Geometry: final body of the model. Coordinates: model frame, mm. Face numbers are marked on the shaded views. A direction names the side the tool comes from. Give positions to 0.01 mm unless a question says otherwise; leave off trailing zeros. Loops run counter-clockwise (first coordinate to the right, second up) from the corner with the lowest first, then second, coordinate; pieces in that order, holes last.
from build123d import *

# Parameters (mm, degrees)
BOSS_EXTRUDE1_START = 1.6
SKETCH2_R           = 4.7625
BOSS_EXTRUDE1_DEPTH = 2.3
BOSS_EXTRUDE2_START = 4.5
SKETCH5_R           = 0.846945363
BOSS_EXTRUDE2_DEPTH = 1
SKETCH6_R           = 0.645187132
CUT_EXTRUDE1_DEPTH  = 5
SKETCH9_W           = 0.137399245
SKETCH9_H           = 0.594121804
BOSS_EXTRUDE3_DEPTH = 3
SKETCH11_R          = 0.94402027
CUT_EXTRUDE2_DEPTH  = 3
SKETCH13_R          = 0.99938664
SKETCH13_R_2        = 0.759397748
CUT_EXTRUDE4_DEPTH  = 4


with BuildPart() as part:
    # Sketch1 → Revolve1 (revolve)
    with BuildSketch(Plane.XY):
        Polygon((0, 7.249356935), (-2.68096621, 7.249356935), (-2.68096621, 0), (-4.484856827, 0), (-4.484856827, 10.8), (-4.7625, 10.8), (-4.7625, 0), (-6.35, 0), (-6.35, -1.2), (-4.7625, -1.2), (-4.7625, -8.33684753), (-4.138651138, -9.1), (-4.138651138, -11.4), (-1.05, -11.4), (-1.05, -13.015612484), (0, -13.015612484), align=None)
    revolve(axis=Axis((0, 72.402332312, 0), (0, -1, 0)))

    # Sketch2 → Boss-Extrude1 (add)
    with BuildSketch(Plane.XZ.offset(1.2).offset(BOSS_EXTRUDE1_START)):
        Polygon((3.666174209, -6.35), (7.332348419, 0), (3.666174209, 6.35), (-3.666174209, 6.35), (-7.332348419, 0), (-3.666174209, -6.35), align=None)
        Circle(SKETCH2_R, mode=Mode.SUBTRACT)
    extrude(amount=BOSS_EXTRUDE1_DEPTH)

    # Sketch4 → Cut-Revolve1 (revolve, cut)
    with BuildSketch(Plane.XY):
        Polygon((-6.925646916, -2.8), (-7.332348419, -3.186501065), (-8.999279983, -3.186501065), (-8.361056601, -0.327260314), (-6.925646916, 0.349979738), align=None)
        Polygon((-6.925646916, -8.249979738), (-6.925646916, -5.1), (-7.332348419, -4.713498935), (-8.999279983, -4.713498935), (-8.361056601, -7.572739686), align=None)
    revolve(axis=Axis((0, 10.8, 0), (0, -1, 0)), mode=Mode.SUBTRACT)

    # Sketch5 → Boss-Extrude2 (add)
    with BuildSketch(Plane.XY.offset(BOSS_EXTRUDE2_START)):
        with Locations((0, 7.245112304)):
            Circle(SKETCH5_R)
    boss_extrude2 = extrude(amount=BOSS_EXTRUDE2_DEPTH)

    # Mirror1: Boss-Extrude2 across plane
    add(boss_extrude2.mirror(Plane.XY))

    # Sketch6 → Cut-Extrude1 (cut)
    with BuildSketch(Plane(origin=(0, 7.249356935, 0), x_dir=(1, 0, 0), z_dir=(0, 1, 0))):
        Circle(SKETCH6_R)
    extrude(amount=-CUT_EXTRUDE1_DEPTH, mode=Mode.SUBTRACT)

    # Sketch9 → Cut-Revolve2 (revolve, cut)
    with BuildSketch(Plane(origin=(0, 0, 0), x_dir=(0, 0, -1), z_dir=(1, 0, 0))):
        with Locations((4.693800378, 8.389118569)):
            Rectangle(SKETCH9_W, SKETCH9_H)
        with Locations((-4.693800378, 8.389118569)):
            Rectangle(SKETCH9_W, SKETCH9_H)
    revolve(axis=Axis((0, 7.245112304, 5.5), (0, 0, -1)), mode=Mode.SUBTRACT)

    # Sketch10 → Boss-Extrude3 (add)
    with BuildSketch(Plane.XZ.offset(13.015612484)):
        with BuildLine():
            Line((0.94402027, 0), (1.05, 0))
            ThreePointArc((1.05, 0), (0, 1.05), (-1.05, 0))
            Line((-1.05, 0), (-0.94402027, 0))
            ThreePointArc((-0.94402027, 0), (0, 0.94402027), (0.94402027, 0))
        make_face()
    extrude(amount=BOSS_EXTRUDE3_DEPTH)

    # Sketch11 → Cut-Extrude2 (cut)
    with BuildSketch(Plane.XZ.offset(13.015612484)):
        Circle(SKETCH11_R)
    extrude(amount=-CUT_EXTRUDE2_DEPTH, mode=Mode.SUBTRACT)

    # Sketch13 → Cut-Extrude4 (cut)
    with BuildSketch(Plane(origin=(0, 7.249356935, 0), x_dir=(1, 0, 0), z_dir=(0, 1, 0))):
        Circle(SKETCH13_R)
        Circle(SKETCH13_R_2, mode=Mode.SUBTRACT)
    extrude(amount=-CUT_EXTRUDE4_DEPTH, mode=Mode.SUBTRACT)


solid = part.part
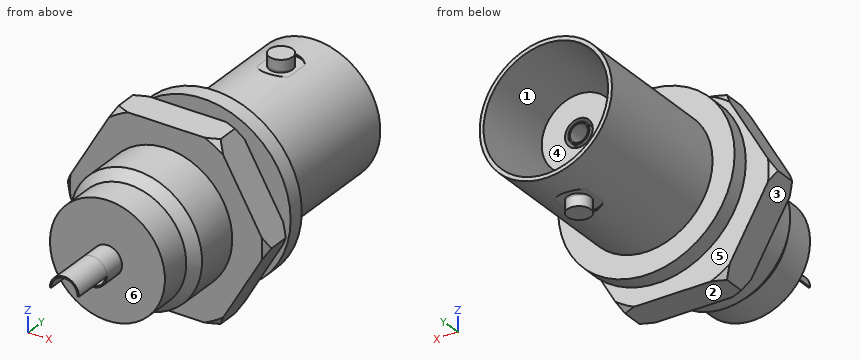
Item 1: Section query C-C on y = -12.25. Return loops of the section in (x, z).
Values follow:
outline: circle Ø2.1 at (0, 0); hole circle Ø1.89 at (0, 0)
Item 2: Section query A-A on y = 3.75. Return loops of the section in (x, z) (1 decimal).
Values follow:
outline: circle Ø9.5 at (0, 0); circle Ø5.4 at (0, 0); circle Ø1.5 at (0, 0); hole circle Ø9 at (0, 0); hole circle Ø2 at (0, 0); hole circle Ø1.3 at (0, 0)
Item 3: Set-up query: the marked faces 4, 5 and 6. Return all of +Z, -Z, +X, -X, +Y, -Y with unobstructed straight access to the full face (end or side cutting, diameter ignored); none if empty.
Values follow:
face 4: +Y
face 5: none
face 6: -Y
Item 4: Pin query (flat end, axial travel): pin 1 (1.5 mm diameter, centred on x = -0.5, y = -7.5, fed in from -Z); pin 2 (0.6 mm diameter, centred on x = 0.5, z = -0.5, fed in from -Y); pin 3 (3 mm diameter, centred on x = -3, y = -9, fed in from +Z); pin 4 (5 mm diameter, centred on x = 5, z = 5, fed in from +Y). Return the tip coordinate at first contact, or that it passes through.
Values follow:
pin 1: stops at z = -4.76
pin 2: stops at y = -13.02
pin 3: stops at z = 4.47
pin 4: stops at y = 10.8
Item 5: Section query D-D on y = 0.5. Return loops of the section in (x, z) (1 decimal), plus the area to 3 significant figures.
Values follow:
outline: circle Ø9.5 at (0, 0); circle Ø5.4 at (0, 0); hole circle Ø9 at (0, 0)
area: 30.6 mm2
Item 6: Section query B-B on x = -5.75. Return loops of the section in (y, z), plus the area to 3 significant figures.
Values follow:
outline: (-5.1, -2.74) - (-2.8, -2.74) - (-2.8, 2.74) - (-5.1, 2.74) - close; (-1.2, -2.69) - (0, -2.69) - (0, 2.69) - (-1.2, 2.69) - close
area: 19.1 mm2
Item 7: Draft query along X for the marked faces 1, 2 and 3. Return one class per face: +X half, -X half, draft (parallel to the pull), parting line (faces both ways), or undercut.
Values follow:
face 1: undercut
face 2: draft
face 3: -X half
Item 8: Ray query, probe 1 along X at (y, z) = (-10.95, 0); probe 2 along Z at (x, y) = (-2.25, 1.5); probe 3 along Y at (x, z) = (-5.5, -1). Return the intervals inside material, ascending.
Values follow:
probe 1: x = -4.14 to -0.94, 0.94 to 4.14
probe 2: z = -4.2 to -3.88, -1.46 to 1.46, 3.88 to 4.2
probe 3: y = -5.1 to -2.8, -1.2 to 0
